The listing builds one solid part. Answer for the finished solid, in the listing's coordinates (mm). A direction names the side the tool comes from. Give positions to 0.01 mm unless a question says otherwise; leave off trailing zeros. Order: outer loops, then holes, each group sorted by start corner. A loop starts at its lowest first (then second) coordinate and runs counter-clockwise, first axis right, second up. Notation, with made-up numbers: (41.25, -38.5) - (99.25, -38.5) arc R9 ccw to (99.25, -32.5) - close; hole circle Ø9 at (11, 10). An arc over 180 degrees is marked (long way). Answer as a JSON object with one key per item and string values. Group by question number.
Q1. For faces 5 (the face through (-14.19, 14.35, 1.67)), 6 (the face through (2.198, -11.537, -4.225)), 7 (the face through (-6.69, -4.96, -0.91)), 8 (the face through (1.5, -9, 10.3)), determine the directions among +Z, -Z, +X, -X, +Y, -Y from which every point of the face is accessible in a straight line to the end or side of a thin tool.
Q2. A cutting plane is placed at D-D, the plane y = -2. Give the vertices of the cut face in (x, z).
Q3. The mould has two halves that part along Y. Classify faces 1 (the face through (25.4, 0, 0)), 2 (the face through (-19, 0, -19)), 3 (the face through (0, -10, -7.62)), 4 (the face through (-11.3, 9.525, -1.2)): released by +Y, released by -Y, zero draft, split by the parting line, or undercut.
Q4. Given pin 1 (1.5 mm diameter, centred on x = -18, z = -20, fed in from -Y); pin 2 (5.5 mm diameter, centred on x = -10.5, z = 1, fed in from +Y) (3 decimals); pin 3 (7.5 mm diameter, centred on x = 0, z = 0, fed in from -Y); pin 4 (4 mm diameter, centred on x = -8.89, z = 0, fed in from +Y), each flat-ended and moving along its own axis, determine where each tip first touches the part or whether it passes through.
Q5. Consider line 1 (Z direction, x = -19.05, y = -12.75); line 2 (Z direction, x = -9, y = -5); line 3 (Y direction, x = 0, z = 20.75). Determine where each line is inside the solid, lowest interval first.
Q6. A cutting plane is placed at C-C, the plane y = 14.5. Give the vertices of the cut face in (x, z).
from build123d import *

# Parameters (mm, degrees)
F0_W      = 50.8
F0_H      = 50.8
F1_DEPTH  = 19.05
F2_R      = 4.7625
F3_DEPTH  = 15.24
F4_R      = 1.5875
F5_DEPTH  = 33.02
F6_R      = 5.55625
F7_DEPTH  = 9.525
F8_R      = 2.38125
F9_DEPTH  = 38.1
F10_R     = 5.55625
F11_DEPTH = 9.525
F12_R     = 2.5527
F13_DEPTH = 19.05


with BuildPart() as f1:
    # F0 (on Front) → F1 (new body, symmetric)
    with BuildSketch(Plane.XZ):
        Rectangle(F0_W, F0_H)
    extrude(amount=F1_DEPTH, both=True)

    # F2 (on face) → F3 (cut)
    with BuildSketch(Plane.XZ.offset(19.05)):
        Circle(F2_R)
    extrude(amount=-F3_DEPTH, mode=Mode.SUBTRACT)

    # F4 (on face) → F5 (cut)
    with BuildSketch(Plane.XY.offset(25.4)):
        with Locations((0, -9.525)):
            Circle(F4_R)
    extrude(amount=-F5_DEPTH, mode=Mode.SUBTRACT)

    # F6 (on face) → F7 (cut)
    with BuildSketch(Plane.XY.offset(25.4)):
        with Locations((0, -9.525)):
            Circle(F6_R)
    extrude(amount=-F7_DEPTH, mode=Mode.SUBTRACT)

    # F8 (on face) → F9 (cut, through all)
    with BuildSketch(Plane.XZ.offset(19.05)):
        with Locations((-8.89, 0)):
            Circle(F8_R)
    extrude(amount=-F9_DEPTH, mode=Mode.SUBTRACT)

    # F10 (on face) → F11 (cut)
    with BuildSketch(Plane(origin=(0, 19.05, 0), x_dir=(-1, 0, 0), z_dir=(0, 1, 0))):
        with Locations((8.89, 0)):
            Circle(F10_R)
    extrude(amount=-F11_DEPTH, mode=Mode.SUBTRACT)

    # F12 (on face) → F13 (cut)
    with BuildSketch(Plane.XZ.offset(19.05)):
        with Locations((-19.05, 19.05)):
            Circle(F12_R)
        with Locations((19.05, 19.05)):
            Circle(F12_R)
        with Locations((-19.05, -19.05)):
            Circle(F12_R)
        with Locations((19.05, -19.05)):
            Circle(F12_R)
    extrude(amount=-F13_DEPTH, mode=Mode.SUBTRACT)


solid = f1.part
Reply:
{
 "1": {"face 5": "+Y", "face 6": "-Y", "face 7": "+Y, -Y", "face 8": "+Z"},
 "2": {"outline": "(-25.4, -25.4) - (25.4, -25.4) - (25.4, 25.4) - (-25.4, 25.4) - close; hole circle Ø5.11 at (-19.05, -19.05); hole circle Ø5.11 at (-19.05, 19.05); hole circle Ø4.76 at (-8.89, 0); hole circle Ø5.11 at (19.05, -19.05); hole circle Ø5.11 at (19.05, 19.05)"},
 "3": {"face 1": "zero draft", "face 2": "released by -Y", "face 3": "undercut", "face 4": "released by +Y"},
 "4": {"pin 1": "stops at y = 0", "pin 2": "stops at y = 9.525", "pin 3": "stops at y = -3.81", "pin 4": "passes through"},
 "5": {"line 1": "z = -25.4 to -21.6, -16.5 to 16.5, 21.6 to 25.4", "line 2": "z = -25.4 to -2.38, 2.38 to 25.4", "line 3": "y = -19.05 to -15.08, -3.97 to 19.05"},
 "6": {"outline": "(-25.4, -25.4) - (25.4, -25.4) - (25.4, 25.4) - (-25.4, 25.4) - close; hole circle Ø11.11 at (-8.89, 0)"}
}
